```python
from build123d import *

# Parameters (mm, degrees)
SKETCH1_W           = 4.78
SKETCH1_H           = 7.6
BOSS_EXTRUDE1_DEPTH = 1.175
DRAFT1_START        = -2.39
DRAFT1_DEPTH        = 4.78
DRAFT1_START_2      = -5
DRAFT1_2_DEPTH      = 10
DRAFT2_START        = -2.39
DRAFT2_DEPTH        = 4.78
DRAFT2_START_2      = -5
DRAFT2_2_DEPTH      = 10
SKETCH2_W           = 0.51
SKETCH2_H           = 0.33
SKETCH5_R           = 0.385012942
CUT_EXTRUDE1_DEPTH  = 0.1


with BuildPart() as part:
    # Sketch1 → Boss-Extrude1 (new, symmetric)
    with BuildSketch(Plane(origin=(0, 0, 0), x_dir=(1, 0, 0), z_dir=(0, 1, 0))):
        Rectangle(SKETCH1_W, SKETCH1_H)
    extrude(amount=BOSS_EXTRUDE1_DEPTH, both=True)

    # Draft1: read off the stored shape, not the designer's step
    # Draft1 outline → Draft1 (cut)
    with BuildSketch(Plane.YZ.offset(DRAFT1_START)):
        Polygon((0, 3.8), (1.175, 3.592815798), (1.175, 3.8), align=None)
        Polygon((1.175, -3.592815798), (0, -3.8), (1.175, -3.8), align=None)
    extrude(amount=DRAFT1_DEPTH, mode=Mode.SUBTRACT)

    # Draft1 2 outline → Draft1 2 (cut)
    with BuildSketch(Plane.XY.offset(DRAFT1_START_2)):
        Polygon((2.39, 1.175), (2.182815798, 1.175), (2.39, 0), align=None)
        Polygon((-2.39, 0), (-2.182815798, 1.175), (-2.39, 1.175), align=None)
    extrude(amount=DRAFT1_2_DEPTH, mode=Mode.SUBTRACT)

    # Draft2: read off the stored shape, not the designer's step
    # Draft2 outline → Draft2 (cut)
    with BuildSketch(Plane.YZ.offset(DRAFT2_START)):
        Polygon((0, -3.8), (-1.175, -3.592815798), (-1.175, -3.8), align=None)
        Polygon((-1.175, 3.592815798), (0, 3.8), (-1.175, 3.8), align=None)
    extrude(amount=DRAFT2_DEPTH, mode=Mode.SUBTRACT)

    # Draft2 2 outline → Draft2 2 (cut)
    with BuildSketch(Plane.XY.offset(DRAFT2_START_2)):
        Polygon((-2.39, -1.175), (-2.182815798, -1.175), (-2.39, 0), align=None)
        Polygon((2.39, 0), (2.182815798, -1.175), (2.39, -1.175), align=None)
    extrude(amount=DRAFT2_2_DEPTH, mode=Mode.SUBTRACT)

    # Sweep1: sweep along a path in Sketch3
    with BuildLine(Plane(origin=(0, 0, 0), x_dir=(0, 0, -1), z_dir=(1, 0, 0))) as sweep1_path:
        Line((-5.2, -1.31), (-4.618685307, -1.31))
        ThreePointArc((-4.618685307, -1.31), (-4.489740009, -1.262882667), (-4.421550295, -1.1437311))
        Line((-4.421550295, -1.1437311), (-4.254300072, -0.1662689))
        ThreePointArc((-4.254300072, -0.1662689), (-4.186110358, -0.047117333), (-4.05716506, 0))
        Line((-4.05716506, 0), (-3.8, 0))
        Line((-3.8, 0), (-2.8, 0))
    # Sketch2 → Sweep1 (sweep)
    with BuildSketch(Plane.XY.offset(3.8)):
        Rectangle(SKETCH2_W, SKETCH2_H)
        with Locations((1.27, 0)):
            Rectangle(SKETCH2_W, SKETCH2_H)
        with Locations((-1.27, 0)):
            Rectangle(SKETCH2_W, SKETCH2_H)
    sweep1 = sweep(path=sweep1_path.line)

    # Mirror1: Sweep1 across plane
    add(sweep1.mirror(Plane.XY))

    # Sketch5 → Cut-Extrude1 (cut)
    with BuildSketch(Plane(origin=(0, 1.175, 0), x_dir=(1, 0, 0), z_dir=(0, 1, 0))):
        with Locations(Location((1.399803613, 2.864403821, 0), (0, 0, 270))):
            Circle(SKETCH5_R)
    extrude(amount=-CUT_EXTRUDE1_DEPTH, mode=Mode.SUBTRACT)


solid = part.part
```
Work out the finished part from the listing and answer in its coordinate system (mm). A direction names the side the tool comes from. Round coordinates to 2 decimals unless told otherwise and drop trailing zeros. Loops run counter-clockwise (first coordinate to the right, second up) from the corner with the lowest first, then second, coordinate; pieces in that order, holes last.
(1) For faces 4 (the flat face through (2.288, -0.579, -0.053)), 5 (the flat face through (0, -1.175, 0)), determine the directions among +Z, -Z, +X, -X, +Y, -Y from which every point of the face is accessible in a straight line to the end or side of a thin tool.
Computed values:
face 4: +Z, -Z, +X, -Y
face 5: +X, -X, -Y
(2) The mould has two halves that part along X. Classify faces 1 (the flat face through (-1.525, -0.83, 4.38)), 2 (the flat face through (0, 1.175, 0)), 3 (the flat face through (-0.255, -0.83, 4.38)): pulls with the +X half, pulls with the -X half, needs draft (parallel to the pull), parting line crosses it, or undercut.
Computed values:
face 1: pulls with the -X half
face 2: needs draft
face 3: undercut
(3) The part is cut by section C-C, the plane z = -1.75. Give the vertices of the cut face in (x, y) (3 decimals).
Computed values:
outline: (-2.39, 0) - (-2.183, -1.175) - (2.183, -1.175) - (2.39, 0) - (2.183, 1.175) - (-2.183, 1.175) - close
(4) The part is cut by section D-D, the plane y = 0.6. Give the vertices of the cut face in (x, z), and give its area (3 significant figures).
Computed values:
outline: (-2.28, -3.69) - (2.28, -3.69) - (2.28, 3.69) - (-2.28, 3.69) - close
area: 33.8 mm2
(5) Find the intervals of material crossed by L1, parallel to X at y = -0.45, z = 4.25 (3 decimals); L2, parallel to Y at x = 0.95, z = -3 (3 decimals); L3, parallel to Z at x = -0.35, y = 0, in increasing order.
Computed values:
L1: x = -1.525 to -1.015, -0.255 to 0.255, 1.015 to 1.525
L2: y = -1.175 to 1.175
L3: z = -3.8 to 3.8
(6) The part is cut by section A-A, the plane x = -1.35. Give the vertices of the cut face in (y, z) (3 decimals), and give its area (3 significant figures).
Computed values:
outline: (-1.475, -5.2) - (-1.145, -5.2) - (-1.145, -4.619) arc R0.035 cw to (-1.116, -4.584) - (-0.138, -4.417) arc R0.365 ccw to (0.165, -4.057) - (0.165, -3.771) - (1.175, -3.593) - (1.175, 3.593) - (0.165, 3.771) - (0.165, 4.057) arc R0.365 ccw to (-0.138, 4.417) - (-1.116, 4.584) arc R0.035 cw to (-1.145, 4.619) - (-1.145, 5.2) - (-1.475, 5.2) - (-1.475, 4.619) arc R0.365 ccw to (-1.172, 4.259) - (-0.194, 4.092) arc R0.035 cw to (-0.165, 4.057) - (-0.165, 3.771) - (-1.175, 3.593) - (-1.175, -3.593) - (-0.165, -3.771) - (-0.165, -4.057) arc R0.035 cw to (-0.194, -4.092) - (-1.172, -4.259) arc R0.365 ccw to (-1.475, -4.619) - close
area: 19.0 mm2
(7) Each of these flat-tipped pins is pushed along its axis until it touches: P1, Ø1.1, axis at y = -1, z = -4.5, coming from the +X side (3 decimals); P2, Ø1.1, axis at y = -0.5, z = -5, coming from the -X side (3 decimals); P3, Ø1, axis at x = 1.5, y = 0.5, coming from the -Z side. Where does it stop, or does it pass through?
Computed values:
P1: stops at x = 1.525
P2: stops at x = -1.525
P3: stops at z = -4.36
(8) The part is cut by section B-B, the plane y = -0.65. Give the vertices of the cut face in (x, z) (3 decimals).
Computed values:
outline: (-2.275, -3.685) - (2.275, -3.685) - (2.275, 3.685) - (-2.275, 3.685) - close; (-1.525, -4.504) - (-1.015, -4.504) - (-1.015, -4.17) - (-1.525, -4.17) - close; (-1.525, 4.17) - (-1.015, 4.17) - (-1.015, 4.504) - (-1.525, 4.504) - close; (-0.255, -4.504) - (0.255, -4.504) - (0.255, -4.17) - (-0.255, -4.17) - close; (-0.255, 4.17) - (0.255, 4.17) - (0.255, 4.504) - (-0.255, 4.504) - close; (1.015, -4.504) - (1.525, -4.504) - (1.525, -4.17) - (1.015, -4.17) - close; (1.015, 4.17) - (1.525, 4.17) - (1.525, 4.504) - (1.015, 4.504) - close
